Check sheet for the modelled part. Datum: model origin and axes. Units: mm. Round coordinates to 2 decimals unless told otherwise and drop trailing zeros. Order: outer loops, then holes, each group sorted by start corner. A loop starts at its lowest first (then second) coordinate and runs counter-clockwise, first axis right, second up.
Q1. Cross-section at B-B on z = -10. Record the cut outline in (x, y) (3 decimals).
Q2. Cross-section at C-C on x = 16. Record the cut outline in (y, z) (3 decimals), then the cut area to 3 significant figures.
Q3. Cross-section at A-A on y = 1.35. Record the cut outline in (x, z) (3 decimals).
Q4. Depth check by flat-ended pin: P1, Ø1.6, axis at x = -6.5, y = 2, coming from the -Z side (3 decimals); P2, Ø1.6, axis at y = 2.5, z = 26, coming from the +X side; P3, Ø1.6, axis at x = -28, y = 2.5, coming from the +Z side. Enter the tip coordinate at first touch or a pass-through.
Q5. Scan lines: probe 1 along X at (y, z) = (2.9, 11) (3 decimals); probe 2 along Z at (x, y) = (-22, 2.4); probe 3 along Z at (x, y) = (3, 0.35) (3 decimals). Record each from-to range of solid material in increasing order.
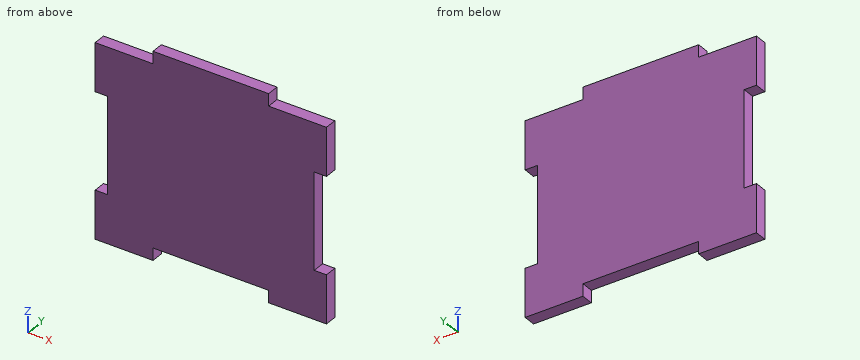
from build123d import *

# Parameters (mm, degrees)
SKETCH1_W           = 60
SKETCH1_H           = 50
BOSS_EXTRUDE1_DEPTH = 3.175
SKETCH2_W           = 30
SKETCH2_H           = 3.175
CUT_EXTRUDE1_DEPTH  = 40.180104964
SKETCH3_W           = 30
SKETCH3_H           = 3.175
BOSS_EXTRUDE2_DEPTH = 3.175
SKETCH5_W           = 3.175
SKETCH5_H           = 25
CUT_EXTRUDE2_DEPTH  = 3.175


with BuildPart() as part:
    # Sketch1 → Boss-Extrude1 (new body)
    with BuildSketch(Plane(origin=(0, 0, 0), x_dir=(1, 0, 0), z_dir=(0, 1, 0))):
        Rectangle(SKETCH1_W, SKETCH1_H)
    extrude(amount=BOSS_EXTRUDE1_DEPTH)

    # Sketch2 → Cut-Extrude1 (cut, through all)
    with BuildSketch(Plane(origin=(0, 3.175, 0), x_dir=(1, 0, 0), z_dir=(0, 1, 0))):
        with Locations((0, 23.4125)):
            Rectangle(SKETCH2_W, SKETCH2_H)
    extrude(amount=-CUT_EXTRUDE1_DEPTH, mode=Mode.SUBTRACT)

    # Sketch3 → Boss-Extrude2 (add)
    with BuildSketch(Plane(origin=(0, 3.175, 0), x_dir=(1, 0, 0), z_dir=(0, 1, 0))):
        with Locations((0, -26.5875)):
            Rectangle(SKETCH3_W, SKETCH3_H)
    extrude(amount=-BOSS_EXTRUDE2_DEPTH)

    # Sketch5 → Cut-Extrude2 (cut)
    with BuildSketch(Plane(origin=(0, 3.175, 0), x_dir=(1, 0, 0), z_dir=(0, 1, 0))):
        with Locations((-28.4125, 0)):
            Rectangle(SKETCH5_W, SKETCH5_H)
        with Locations((28.4125, 0)):
            Rectangle(SKETCH5_W, SKETCH5_H)
    extrude(amount=-CUT_EXTRUDE2_DEPTH, mode=Mode.SUBTRACT)


solid = part.part
Results found:
1. outline: (-26.825, 0) - (26.825, 0) - (26.825, 3.175) - (-26.825, 3.175) - close
2. outline: (0, -25) - (3.175, -25) - (3.175, 25) - (0, 25) - close
2. area: 159 mm2
3. outline: (-30, -25) - (-15, -25) - (-15, -21.825) - (15, -21.825) - (15, -25) - (30, -25) - (30, -12.5) - (26.825, -12.5) - (26.825, 12.5) - (30, 12.5) - (30, 25) - (15, 25) - (15, 28.175) - (-15, 28.175) - (-15, 25) - (-30, 25) - (-30, 12.5) - (-26.825, 12.5) - (-26.825, -12.5) - (-30, -12.5) - close
4. P1: stops at z = -21.825
4. P2: stops at x = 15
4. P3: stops at z = 25
5. probe 1: x = -26.825 to 26.825
5. probe 2: z = -25 to 25
5. probe 3: z = -21.825 to 28.175
